Work out the finished part from the listing and answer in its coordinate system (mm). Face numbers are marked on the shaded views. A direction names the side the tool comes from. Round coordinates to 2 decimals unless told otherwise and drop trailing zeros. Loops run counter-clockwise (first coordinate to the right, second up) from the corner with the lowest first, then second, coordinate; pieces in that order, holes last. Notation, with made-up numbers: (28.25, -26.75) - (61.25, -26.75) arc R20 ccw to (61.25, -16.75) - close; hole circle Ø11 at (-38, -29.75). An arc over 180 degrees is marked (long way). Return JSON: item names as keys, results as strings.
Autodesk Inventor part; units mm, degrees
ref_plane "YZ Plane" through (0, 0, 0) normal (1, 0, 0) x (0, 1, 0)
ref_plane "XZ Plane" through (0, 0, 0) normal (0, 1, 0) x (-1, 0, 0)
ref_plane "XY Plane" through (0, 0, 0) normal (0, 0, 1) x (1, 0, 0)
sketch "草圖1" plane through (0, 0, 0) normal (0, 1, 0) x (-1, 0, 0)
  line L0 (2.5, 5) -> (-2.5, 5)
  line L1 (-2.5, 5) -> (-2.5, -5)
  line L2 (-2.5, -5) -> (2.5, -5)
  line L3 (2.5, -5) -> (2.5, 5)
  circle A0 centre (0, 2.5) radius 1.7
  line L4 (2.5, 0) -> (-2.5, 0) construction
  circle A1 centre (0, -2.5) radius 1.7
  point P0 (0, 0)
  point P1 (0, 5)
  dimension "d0" = 5
  dimension "d1" = 10
  dimension "d2" = 3.4
  dimension "d3" = 2.5
  dimension "d4" = 2.5
extrude "擠出1" add sketch "草圖1" along normal blind 1.6 contours L3 L2 L1 L0 | A0 | A1
extrude "擠出2" cut sketch "草圖1" along normal blind 1.5 contours A0 | A1
extrude "擠出3" cut sketch "草圖1" along normal blind 1.5 contours A0 | A1
properties part number "110033226_ipt_12_平滑面(2x1)"
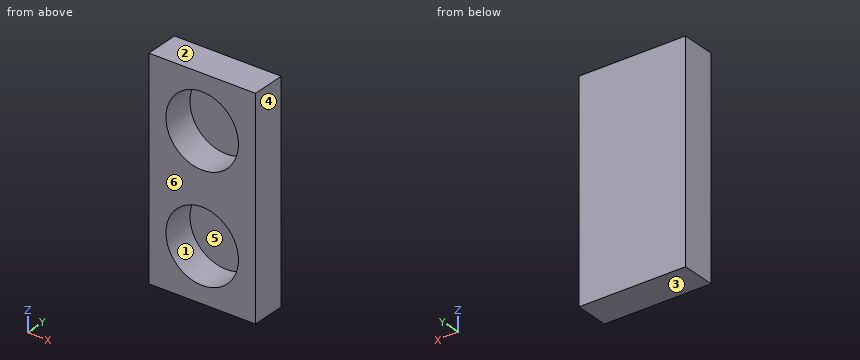
1) Section B-B (x = 0) is taken. Give the vertices of the cut face in (y, z).
Verdict:
{"outline": "(0, -5) - (1.6, -5) - (1.6, 5) - (0, 5) - (0, 4.2) - (1.5, 4.2) - (1.5, 0.8) - (0, 0.8) - (0, -0.8) - (1.5, -0.8) - (1.5, -4.2) - (0, -4.2) - close"}
2) Find the intervals of material crossed by L1, parallel to Z at x = 0, y = 0.85; L2, parallel to Z at x = 1.55, y = 0.4; L3, parallel to X at y = 0.85, z = 2.75, in increasing order.
Verdict:
{"L1": "z = -5 to -4.2, -0.8 to 0.8, 4.2 to 5", "L2": "z = -5 to -3.2, -1.8 to 1.8, 3.2 to 5", "L3": "x = -2.5 to -1.68, 1.68 to 2.5"}
3) A tool of negligible diameter and unlimited length cuts with its end or side. For the marked faces 5 and 6, from which of +Z, -Z, +X, -X, +Y, -Y can it reach the whole face along a straight path? Write none if from no direction.
Verdict:
{"face 5": "-Y", "face 6": "+Z, -Z, +X, -X, -Y"}
4) Section A-A (z = 2.5) is taken. Give the vertices of the cut face in (x, y), and give its area (3 significant figures).
Verdict:
{"outline": "(-2.5, 0) - (-1.7, 0) - (-1.7, 1.5) - (1.7, 1.5) - (1.7, 0) - (2.5, 0) - (2.5, 1.6) - (-2.5, 1.6) - close", "area": "2.90 mm2"}
5) Section D-D (x = 0.8) is taken. Give the vertices of the cut face in (y, z), and give its area (3 significant figures).
Verdict:
{"outline": "(0, -5) - (1.6, -5) - (1.6, 5) - (0, 5) - (0, 4) - (1.5, 4) - (1.5, 1) - (0, 1) - (0, -1) - (1.5, -1) - (1.5, -4) - (0, -4) - close", "area": "7.00 mm2"}
6) A flat-ended cylindrical pin translates along its axis: pin 1 (2.5 mm diameter, centred on x = 0, z = -2.5, fed in from -Y). Find the tip coordinate at first contact, or state that the pin passes through.
Verdict:
{"pin 1": "stops at y = 1.5"}
7) Section C-C (y = 1.3) is taken. Give the vertices of the cut face in (x, z), and give its area (3 significant figures).
Verdict:
{"outline": "(-2.5, -5) - (2.5, -5) - (2.5, 5) - (-2.5, 5) - close; hole circle Ø3.4 at (0, -2.5); hole circle Ø3.4 at (0, 2.5)", "area": "31.8 mm2"}
8) Determine the mould class of the marked faces 1, 2, 3 and 4 for opening direction Z: pulls with the +Z half, pulls with the -Z half, needs draft (parallel to the pull), parting line crosses it, or undercut.
Verdict:
{"face 1": "undercut", "face 2": "pulls with the +Z half", "face 3": "pulls with the -Z half", "face 4": "needs draft"}
